The model under review builds one solid part; all positions refer to its coordinate system, in mm. A direction names the side the tool comes from. Round coordinates to 2 decimals unless told otherwise and drop trailing zeros. Write each loop counter-clockwise with the first axis right and the second up, starting at its lowest first coordinate (ties: lowest second). Pieces come first, ordered by that corner, then holes.
Item 1: Add section D-D (y = 33). Give the boundary of the cut face in (x, z), plus the area to 3 significant figures.
Item 2: Add section A-A (y = -5). Give the boundary of the cut face in (x, z), plus the area to 4 significant figures.
Item 3: Machinability: for faces 1 (the face through (-11, 30, 7)), 2 (the face through (25.5, 3, 1)), 3 (the face through (-0.2, -18, 8.4)), which of the approach directions +Z, -Z, +X, -X, +Y, -Y give a long, thin tool a straight path to every point of the face, cutting with its end or side? Answer none if there is none.
Item 4: Clearance check with flat-ended pins moving along their axes: pin 1 Ø1.1 at (y, z) = (1, 0.5) entering from -X; pin 2 Ø2.5 at (x, y) = (14, -16.5) entering from +Z; pin 3 Ø14 at (x, y) = (-4.5, 3.5) entering from +Z. State where each tip first meets the part, or that it passes through.
Item 5: Add section C-C (x = -14.5). Give the boundary of the cut face in (y, z).
Item 6: To check wall thickness, follow L1, parallel to Y at x = -6.5, z = 5; L2, parallel to X at y = 36.5, z = 3; L3, parallel to X at y = 20, z = 2.25. State the ranges of each line that lie inside material, in increasing order.
Item 7: Draft analysis for pull direction X (two halves, no side actions). For faces 4 (the face through (-24, 4, 2.5)), 5 (the face through (-10.08, 30.05, 4.46)), 6 (the face through (24.268, 20.598, 1.232)), state which applies: +X half, -X half, draft (parallel to the pull), parting line (faces both ways), or undercut.
Item 8: Add section B-B (z = 6.25). Give the boundary of the cut face in (x, y).
```python
from build123d import *

# Parameters (mm, degrees)
PAD_DEPTH       = 2
POCKET_DEPTH    = 1
SKETCH002_W     = 4.5
SKETCH002_H     = 11.5
POCKET001_DEPTH = 5
SKETCH003_W     = 8
SKETCH003_H     = 1.5
PAD001_DEPTH    = 1
SKETCH004_W     = 26
SKETCH004_H     = 2
PAD002_DEPTH    = 9
SKETCH005_W     = 20
SKETCH005_H     = 2
PAD003_DEPTH    = 6
SKETCH006_W     = 3
SKETCH006_H     = 7
PAD004_DEPTH    = 3
PAD005_DEPTH    = 2.5
SKETCH008_W     = 17
SKETCH008_H     = 1
PAD006_DEPTH    = 0.5
PAD008_DEPTH    = 0.5
SKETCH013_W     = 2.0000000001
SKETCH013_H     = 3
PAD009_DEPTH    = 5
POCKET002_DEPTH = 20
POCKET003_DEPTH = 20


with BuildPart() as part:
    # Sketch → Pad (new body)
    with BuildSketch(Plane.XY):
        Polygon((-25, -20), (25, -20), (25, 20), (0, 40), (-25, 20), align=None)
    extrude(amount=PAD_DEPTH)

    # Sketch001 → Pocket (cut)
    with BuildSketch(Plane.XY.offset(2)):
        with BuildLine():
            Line((-3, 15), (3, 15))
            Line((3, 15), (3, 21))
            ThreePointArc((3, 21), (0, 21.8038475773), (-3, 21))
            Line((-3, 15), (-3, 21))
        make_face()
        with BuildLine():
            Line((-6, -16), (6, -16))
            Line((6, -16), (6, 2))
            ThreePointArc((6, 2), (0, 3.1676030258), (-6, 2))
            Line((-6, -16), (-6, 2))
        make_face()
    extrude(amount=-POCKET_DEPTH, mode=Mode.SUBTRACT)

    # Sketch002 → Pocket001 (cut)
    with BuildSketch(Plane.XY.offset(1)):
        with BuildLine():
            Line((-2, 16), (2, 16))
            Line((2, 16), (2, 20))
            ThreePointArc((2, 20), (0, 20.5358983849), (-2, 20))
            Line((-2, 16), (-2, 20))
        make_face()
        with Locations((-2.75, -6.25)):
            Rectangle(SKETCH002_W, SKETCH002_H)
        with Locations((2.75, -6.25)):
            Rectangle(SKETCH002_W, SKETCH002_H)
        with BuildLine():
            Line((-5, 0.5), (-0.5, 0.5))
            Line((-0.5, 0.5), (-0.5, 2))
            ThreePointArc((-0.5, 2), (-2.7826111414, 1.7479786314), (-5, 1.1504712732))
            Line((-5, 0.5), (-5, 1.1504712732))
        make_face()
        with BuildLine():
            Line((0.5, 0.5), (5, 0.5))
            Line((5, 0.5), (5, 1.1504712732))
            ThreePointArc((5, 1.1504712732), (2.7826111414, 1.7479786314), (0.5, 2))
            Line((0.5, 0.5), (0.5, 2))
        make_face()
    extrude(amount=-POCKET001_DEPTH, mode=Mode.SUBTRACT)

    # Sketch003 → Pad001 (new body)
    with BuildSketch(Plane.XY.offset(2)):
        with Locations((0, 14.25)):
            Rectangle(SKETCH003_W, SKETCH003_H)
    extrude(amount=PAD001_DEPTH)

    # Sketch004 → Pad002 (new body)
    with BuildSketch(Plane.XY.offset(2)):
        with Locations((0, -19)):
            Rectangle(SKETCH004_W, SKETCH004_H)
    extrude(amount=PAD002_DEPTH)

    # Sketch005 → Pad003 (new body)
    with BuildSketch(Plane.XY.offset(2)):
        with Locations((0, -17)):
            Rectangle(SKETCH005_W, SKETCH005_H)
    extrude(amount=PAD003_DEPTH)

    # Sketch006 → Pad004 (new body)
    with BuildSketch(Plane(origin=(0, 0, 0), x_dir=(1, 0, 0), z_dir=(0, 0, -1))):
        with Locations((-24.5, 16.5)):
            Rectangle(SKETCH006_W, SKETCH006_H)
        with Locations((24.5, 16.5)):
            Rectangle(SKETCH006_W, SKETCH006_H)
    extrude(amount=-PAD004_DEPTH)

    # Sketch007 → Pad005 (new body)
    with BuildSketch(Plane(origin=(0, 0, 0), x_dir=(1, 0, 0), z_dir=(0, 0, -1))):
        Polygon((-25.5, 20), (-23, 20), (-23, -21.624460083), (-25.5, -19.6), align=None)
        Polygon((23, 20), (25.5, 20), (25.5, -19.6), (23, -21.624460083), align=None)
    extrude(amount=-PAD005_DEPTH)

    # Sketch008 → Pad006 (new body)
    with BuildSketch(Plane.XY.offset(2)):
        with Locations((-14.5, -14.5)):
            Rectangle(SKETCH008_W, SKETCH008_H)
        with Locations((14.5, -14.5)):
            Rectangle(SKETCH008_W, SKETCH008_H)
    extrude(amount=PAD006_DEPTH)

    # Sketch012 → Pad008 (new body)
    with BuildSketch(Plane.XY.offset(2)):
        with BuildLine():
            ThreePointArc((3, 21), (0, 21.8309518948), (-3, 21))
            Line((-3, 21), (-3, 15))
            Line((-3.75, 15), (-3, 15))
            Line((-3.75, 21.6561501911), (-3.75, 15))
            Line((-3.3030993045, 21.6561501911), (-3.75, 21.6561501911))
            ThreePointArc((3.3030993045, 21.6561501911), (0, 22.55), (-3.3030993046, 21.6561501911))
            Line((3.3030993045, 21.6561501911), (3.75, 21.6561501911))
            Line((3.75, 21.6561501911), (3.75, 15))
            Line((3.75, 15), (3, 15))
            Line((3, 15), (3, 21))
        make_face()
        with BuildLine():
            Line((-6, 2), (-6, -16))
            Line((-6, -16), (-6.75, -16))
            Line((-6.75, -16), (-6.75, 3.1718383847))
            Line((-6.75, 3.1718383847), (-6.1651012574, 3.1718383847))
            ThreePointArc((6.1651012573, 3.1718383847), (0, 4.3182305052), (-6.1651012574, 3.1718383847))
            Line((6.1651012574, 3.1718383847), (6.75, 3.1718383847))
            Line((6.75, 3.1718383847), (6.75, -16))
            Line((6, -16), (6.75, -16))
            Line((6, -16), (6, 2))
            ThreePointArc((6, 2), (0, 3.1676030258), (-6, 2))
        make_face()
    extrude(amount=PAD008_DEPTH)

    # Sketch013 → Pad009 (new body)
    with BuildSketch(Plane.XY.offset(2)):
        with Locations((0, 37.7)):
            Rectangle(SKETCH013_W, SKETCH013_H)
        Polygon((-11, 31.2), (-9.1259148573, 28.8573935717), (-10.2972180715, 27.9203510003), (-12.1713032142, 30.2629574287), align=None)
        Polygon((-21.8286967858, 22.5370425713), (-19.9546116432, 20.194436143), (-21.1259148573, 19.2573935717), (-23, 21.6), align=None)
        Polygon((19.9546116432, 20.194436143), (21.8286967858, 22.5370425713), (23, 21.6), (21.1259148573, 19.2573935717), align=None)
        Polygon((11, 31.2), (12.1713032142, 30.2629574287), (10.2972180715, 27.9203510003), (9.1259148573, 28.8573935717), align=None)
    extrude(amount=PAD009_DEPTH)

    # Sketch014 → Pocket002 (cut)
    with BuildSketch(Plane(origin=(-3.4878048781, -2.7902439024, 0), x_dir=(0.6246950476, -0.7808688094, 0), z_dir=(-0.7808688094, -0.6246950476, 0))):
        Polygon((-29.2347523777, 7), (-28.2347523777, 7), (-28.2347523777, 3.5), align=None)
    extrude(amount=-POCKET002_DEPTH, mode=Mode.SUBTRACT)

    # Sketch015 → Pocket003 (cut)
    with BuildSketch(Plane(origin=(3.4878048781, -2.7902439024, 0), x_dir=(0.6246950476, 0.7808688094, 0), z_dir=(0.7808688094, -0.6246950476, 0))):
        Polygon((28.2347523777, 7), (28.2347523777, 3.5), (29.2347523777, 7), align=None)
    extrude(amount=-POCKET003_DEPTH, mode=Mode.SUBTRACT)


solid = part.part
```
Numbers:
1. outline: (-8.75, 0) - (8.75, 0) - (8.75, 2) - (-8.75, 2) - close
1. area: 35.0 mm2
2. outline: (-25.5, 0) - (-5, 0) - (-5, 1) - (-6, 1) - (-6, 2.5) - (-6.75, 2.5) - (-6.75, 2) - (-23, 2) - (-23, 2.5) - (-25.5, 2.5) - close; (-0.5, 0) - (0.5, 0) - (0.5, 1) - (-0.5, 1) - close; (5, 0) - (25.5, 0) - (25.5, 2.5) - (23, 2.5) - (23, 2) - (6.75, 2) - (6.75, 2.5) - (6, 2.5) - (6, 1) - (5, 1) - close
2. area: 84.25 mm2
3. face 1: +Z, +X, -X, +Y
3. face 2: +Z, -Z, +X, +Y
3. face 3: +Z
4. pin 1: stops at x = -25.5
4. pin 2: stops at z = 2
4. pin 3: stops at z = 2.5
5. outline: (-20, 0) - (28.4, 0) - (28.4, 2) - (-14, 2) - (-14, 2.5) - (-15, 2.5) - (-15, 2) - (-20, 2) - close
6. L1: y = -20 to -16
6. L2: x = -1 to 1
6. L3: x = -25.01 to -23, -21.72 to -20.2, -3.75 to -3, 3 to 3.75, 20.2 to 21.72, 23 to 25.01
7. face 4: draft
7. face 5: undercut
7. face 6: +X half
8. outline: (-23, 21.6) - (-21.62, 19.87) - (-20.45, 20.81) - (-21.83, 22.54) - close; (-13, -20) - (13, -20) - (13, -18) - (10, -18) - (10, -16) - (-10, -16) - (-10, -18) - (-13, -18) - close; (-12.17, 30.26) - (-10.79, 28.53) - (-9.62, 29.47) - (-11, 31.2) - close; (-1, 36.2) - (1, 36.2) - (1, 39.2) - (-1, 39.2) - close; (9.62, 29.47) - (10.79, 28.53) - (12.17, 30.26) - (11, 31.2) - close; (20.45, 20.81) - (21.62, 19.87) - (23, 21.6) - (21.83, 22.54) - close
